from build123d import *

# Parameters (mm, degrees)
BOSS_EXTRUDE1_DEPTH = 40
CUT_EXTRUDE1_REACH  = 52.121
SKETCH2_R           = 1.75


with BuildPart() as part:
    # Sketch1 → Boss-Extrude1 (new body)
    with BuildSketch(Plane(origin=(0, 0, 0), x_dir=(0, 1, 0), z_dir=(0, 0, 1))):
        with BuildLine():
            Line((1, 12.760877713), (1, 27.8))
            Line((1, 27.8), (5, 27.8))
            Line((5, 27.8), (5, 16.038703189))
            ThreePointArc((5, 16.038703189), (16.8, 0), (5, -16.038703189))
            Line((5, -16.038703189), (5, -27.760877713))
            Line((5, -27.760877713), (1, -27.760877713))
            Line((1, -27.760877713), (1, -12.760877713))
            ThreePointArc((1, -12.760877713), (12.8, 0), (1, 12.760877713))
        make_face()
    extrude(amount=BOSS_EXTRUDE1_DEPTH)

    # Sketch2 → Cut-Extrude1 (cut, up to next)
    with BuildSketch(Plane(origin=(0, 5, 0), x_dir=(-1, 0, 0), z_dir=(0, 1, 0)), mode=Mode.PRIVATE) as cut_extrude1_sk1:
        with Locations((-22.260877713, 32.5)):
            Circle(SKETCH2_R)
    cut_extrude1_tool1 = extrude(cut_extrude1_sk1.sketch, amount=-CUT_EXTRUDE1_REACH, mode=Mode.PRIVATE) & part.part
    # Sketch2 → Cut-Extrude1 (cut, up to next)
    with BuildSketch(Plane(origin=(0, 5, 0), x_dir=(-1, 0, 0), z_dir=(0, 1, 0)), mode=Mode.PRIVATE) as cut_extrude1_sk2:
        with Locations((-22.260877713, 7.5)):
            Circle(SKETCH2_R)
    cut_extrude1_tool2 = extrude(cut_extrude1_sk2.sketch, amount=-CUT_EXTRUDE1_REACH, mode=Mode.PRIVATE) & part.part
    # Sketch2 → Cut-Extrude1 (cut, up to next)
    with BuildSketch(Plane(origin=(0, 5, 0), x_dir=(-1, 0, 0), z_dir=(0, 1, 0)), mode=Mode.PRIVATE) as cut_extrude1_sk3:
        with Locations(Location((22.260877713, 7.5, 0), (0, 0, 90))):
            Circle(SKETCH2_R)
    cut_extrude1_tool3 = extrude(cut_extrude1_sk3.sketch, amount=-CUT_EXTRUDE1_REACH, mode=Mode.PRIVATE) & part.part
    # Sketch2 → Cut-Extrude1 (cut, up to next)
    with BuildSketch(Plane(origin=(0, 5, 0), x_dir=(-1, 0, 0), z_dir=(0, 1, 0)), mode=Mode.PRIVATE) as cut_extrude1_sk4:
        with Locations(Location((22.260877713, 32.5, 0), (0, 0, 90))):
            Circle(SKETCH2_R)
    cut_extrude1_tool4 = extrude(cut_extrude1_sk4.sketch, amount=-CUT_EXTRUDE1_REACH, mode=Mode.PRIVATE) & part.part
    add(cut_extrude1_tool1.solids().sort_by_distance((22.260878, 5, 32.5))[0], mode=Mode.SUBTRACT)
    add(cut_extrude1_tool2.solids().sort_by_distance((22.260878, 5, 7.5))[0], mode=Mode.SUBTRACT)
    add(cut_extrude1_tool3.solids().sort_by_distance((-22.260878, 5, 7.5))[0], mode=Mode.SUBTRACT)
    add(cut_extrude1_tool4.solids().sort_by_distance((-22.260878, 5, 32.5))[0], mode=Mode.SUBTRACT)


solid = part.part
Can you work these out from the model? Positions are in its coordinate system, mm. A direction names the side the tool comes from. Give positions to 0.01 mm unless a question says otherwise; leave off trailing zeros. Loops run counter-clockwise (first coordinate to the right, second up) from the corner with the lowest first, then second, coordinate; pieces in that order, holes last. Notation, with made-up numbers: (86, 63) -> (134, 63) arc R14 cw to (134, 68) -> close; hole circle Ø9 at (12.5, 34). An arc over 180 degrees is marked (long way). Use one line per item in the form item = value.
1) For faces 1 (the face through (-22, 5, 20)), 2 (the face through (-27.8, 3, 20)), which set-ups out of +Z, -Z, +X, -X, +Y, -Y let a thin tool reach every point of the face, with its end or its side?
Answers:
face_1 = +Z, -Z, -X, +Y
face_2 = +Z, -Z, -X, +Y, -Y
2) If we section it at C-C (y = 6): Please give me the cut outline in (x, z).
Answers:
outline = (-15.69, 0) -> (-11.31, 0) -> (-11.31, 40) -> (-15.69, 40) -> close; (11.31, 0) -> (15.69, 0) -> (15.69, 40) -> (11.31, 40) -> close
3) We'd pull the mould along Z, two halves only. Please class faces 3 (the face through (22, 5, 20)), 4 (the face through (-23.81, 3.03, 8.31)), 5 (the face through (2, 13, 0)): released by +Z, released by -Z, zero draft, split by the parting line, or undercut.
Answers:
face_3 = zero draft
face_4 = undercut
face_5 = released by -Z
4) I need wall thicknesses on line 1 along X through (y, z) = (3, 38.5); line 2 along X through (y, z) = (6.75, 18); line 3 along Y through (x, z) = (18.5, 7). Which ranges of each line are inside material? Lowest first, please.
Answers:
line_1 = -27.8 to -12.44, 12.44 to 27.76
line_2 = -15.38 to -10.88, 10.88 to 15.38
line_3 = 1 to 5
5) If we section it at B-B (y = 3.5): Please give me the cut outline in (x, z), plus the area to 3 significant figures.
Answers:
outline = (-27.8, 0) -> (-12.31, 0) -> (-12.31, 40) -> (-27.8, 40) -> close; (12.31, 0) -> (27.76, 0) -> (27.76, 40) -> (12.31, 40) -> close; hole circle Ø3.5 at (-22.26, 7.5); hole circle Ø3.5 at (-22.26, 32.5); hole circle Ø3.5 at (22.26, 7.5); hole circle Ø3.5 at (22.26, 32.5)
area = 1,200 mm²
6) Will these pins go through, and if not, where does the flat tip stop? pin 1 (2 mm diameter, centred on y = 9.5, z = 16, fed in from -X); pin 2 (13 mm diameter, centred on x = -20, z = 24, fed in from +Y); pin 3 (1 mm diameter, centred on x = 4.5, z = 23, fed in from +Y).
Answers:
pin_1 = -14.49
pin_2 = 10
pin_3 = 16.32
7) If we section it at A-A (z = 7.5): Please give me the cut outline in (x, y).
Answers:
outline = (-27.8, 1) -> (-24.01, 1) -> (-24.01, 5) -> (-27.8, 5) -> close; (-20.51, 1) -> (-12.76, 1) arc R12.8 cw to (12.76, 1) -> (20.51, 1) -> (20.51, 5) -> (16.04, 5) arc R16.8 ccw to (-16.04, 5) -> (-20.51, 5) -> close; (24.01, 1) -> (27.76, 1) -> (27.76, 5) -> (24.01, 5) -> close
8) If we section it at D-D (z = 33.5): Please give me the cut outline in (x, y).
Answers:
outline = (-27.8, 1) -> (-23.7, 1) -> (-23.7, 5) -> (-27.8, 5) -> close; (-20.82, 1) -> (-12.76, 1) arc R12.8 cw to (12.76, 1) -> (20.82, 1) -> (20.82, 5) -> (16.04, 5) arc R16.8 ccw to (-16.04, 5) -> (-20.82, 5) -> close; (23.7, 1) -> (27.76, 1) -> (27.76, 5) -> (23.7, 5) -> close
